Design review of the part built by this model. Coordinates are the model's own, in mm. A direction names the side the tool comes from. Give positions to 0.01 mm unless a question says otherwise; leave off trailing zeros. Write each loop counter-clockwise with the first axis right and the second up, starting at its lowest first coordinate (ties: lowest second). Pieces come first, ordered by that corner, then holes. Notation, with made-up numbers: (73, -27.5) -> (117, -27.5) arc R19 cw to (117, -1.5) -> close; hole circle Ø4 at (-38.5, 15). An arc over 180 degrees is marked (long way). Answer as a JSON object with one key per item and string values.
```python
from build123d import *

# Parameters (mm, degrees)
BASE_FLANGE1_DEPTH   = 3.175
M6_CLEARANCE_HOLE1_D = 6.6
FILLET1_R            = 2.54


# Sheet-metal steps are written as plain solids
with BuildPart() as part:
    # Sketch1 → Base-Flange1 (new body)
    with BuildSketch(Plane.XY):
        Polygon((47.801569048, -78.501600001), (-22.7939, -78.501600001), (-22.7939, -62.123600001), (64.179569048, -62.123600001), (64.179569048, -112.791600001), (47.801569048, -112.791600001), align=None)
    extrude(amount=-BASE_FLANGE1_DEPTH)

    # M6 Clearance Hole1 (through all)
    with Locations(Plane.XY):
        with Locations((56.565919048, -102.268610498), (-14.4119, -70.312600001)):
            Hole(M6_CLEARANCE_HOLE1_D / 2)

    # Fillet1
    fillet1_edges = [part.edges().sort_by_distance(p)[0] for p in [
        (-22.7939, -62.123600001, -1.5875),
        (64.179569048, -62.123600001, -1.5875),
        (64.179569048, -112.791600001, -1.5875),
        (47.801569048, -112.791600001, -1.5875),
        (47.801569048, -78.501600001, -1.5875),
        (-22.7939, -78.501600001, -1.5875),
    ]]
    fillet(fillet1_edges, radius=FILLET1_R)


solid = part.part
```
(1) Clearance check with flat-ended pins moving along their axes: pin 1 (5.5 mm diameter, centred on x = -14.41, y = -70.31, fed in from +Z); pin 2 (1 mm diameter, centred on x = 25.5, z = -2.5, fed in from -Y); pin 3 (1 mm diameter, centred on y = -95.5, z = -1.5, fed in from -X). State where each tip first meets the part, or that it passes through.
Here are the results:
{"pin 1": "passes through", "pin 2": "stops at y = -78.5", "pin 3": "stops at x = 47.8"}
(2) The part is to be moulded in two halves that separate along Y. For faces 3 (the cylindrical face through (48.5, -112, -1.6)), 4 (the cylindrical face through (-16.186, -67.53, -1.61)), 5 (the flat face through (20, -62.124, -2)), 6 (the flat face through (31, -76, -3.175)), say which applies: +Y half, -Y half, draft (parallel to the pull), parting line (faces both ways), or undercut.
Here are the results:
{"face 3": "-Y half", "face 4": "undercut", "face 5": "+Y half", "face 6": "draft"}
(3) We need section B-B, the plane y = -91. State the section outline as (x, z) points (3 decimals), then the cut area to 3 significant figures.
Here are the results:
{"outline": "(47.802, -3.175) -> (64.18, -3.175) -> (64.18, 0) -> (47.802, 0) -> close", "area": "52.0 mm²"}
(4) We need section C-C, the plane x = 12.5. State the section outline as (y, z) points (3 decimals), then the cut area to 3 significant figures.
Here are the results:
{"outline": "(-78.502, -3.175) -> (-62.124, -3.175) -> (-62.124, 0) -> (-78.502, 0) -> close", "area": "52.0 mm²"}
(5) For line 1 along X through (y, z) = (-102.5, -0.6); line 2 along X through (y, z) = (-108, -0.15); line 3 along Y through (x, z) = (37.5, -2.15), list the stretches that pass through material, from the lowest coordinate up.
Here are the results:
{"line 1": "x = 47.8 to 53.27, 59.86 to 64.18", "line 2": "x = 47.8 to 64.18", "line 3": "y = -78.5 to -62.12"}
(6) For faces 1 (the flat face through (56, -112.792, -2)), 2 (the flat face through (13, -78.502, -2)), list the 3-axis set-ups (+Z, -Z, +X, -X, +Y, -Y) from which the entire face can be reached by the end or side of a thin tool; tool diameter is ignored.
Here are the results:
{"face 1": "+Z, -Z, +X, -X, -Y", "face 2": "+Z, -Z, -X, -Y"}
(7) We need section A-A, the plane z = -2.6. State the section outline as (x, y) points.
Here are the results:
{"outline": "(-22.79, -75.96) arc R2.54 ccw to (-20.25, -78.5) -> (45.26, -78.5) arc R2.54 cw to (47.8, -81.04) -> (47.8, -110.25) arc R2.54 ccw to (50.34, -112.79) -> (61.64, -112.79) arc R2.54 ccw to (64.18, -110.25) -> (64.18, -64.66) arc R2.54 ccw to (61.64, -62.12) -> (-20.25, -62.12) arc R2.54 ccw to (-22.79, -64.66) -> close; hole circle Ø6.6 at (-14.41, -70.31); hole circle Ø6.6 at (56.57, -102.27)"}
